Autodesk Inventor part; units mm, degrees
ref_plane "YZ Plane" through (0, 0, 0) normal (1, 0, 0) x (0, 1, 0)
ref_plane "XZ Plane" through (0, 0, 0) normal (0, 1, 0) x (-1, 0, 0)
ref_plane "XY Plane" through (0, 0, 0) normal (0, 0, 1) x (1, 0, 0)
sketch "Sketch1" plane through (0, 0, 0) normal (0, 1, 0) x (-1, 0, 0)
  line L0 (35, 25) -> (-35, 25)
  line L1 (-35, 25) -> (-35, -25)
  line L2 (-35, -25) -> (35, -25)
  line L3 (35, -25) -> (35, 25)
  line L4 (35, 25) -> (-35, -25) construction
  line L5 (-35, 25) -> (35, -25) construction
  line L6 (40, -20) -> (35, -20)
  line L7 (35, -20) -> (35, 20)
  line L8 (35, 20) -> (40, 20)
  line L9 (40, 20) -> (40, -20)
  line L10 (40, -20) -> (35, 20) construction
  line L11 (35, -20) -> (40, 20) construction
  line L12 (-35, -20) -> (-40, -20)
  line L13 (-40, -20) -> (-40, 20)
  line L14 (-40, 20) -> (-35, 20)
  line L15 (-35, 20) -> (-35, -20)
  line L16 (-35, -20) -> (-40, 20) construction
  line L17 (-40, -20) -> (-35, 20) construction
  line L18 (35, 0) -> (0, 0)
  line L19 (37.5, 0) -> (40, 0) construction
  line L20 (-37.5, 0) -> (-35, 0) construction
  point P0 (35, -20)
  point P1 (-35, 20)
  point P2 (-35, -20)
  dimension "d0" = 5
  dimension "d1" = 5
  dimension "d2" = 40
  dimension "d3" = 50
  dimension "d4" = 40
  dimension "d5" = 70
extrude "Extrusion1" add sketch "Sketch1" along normal blind 5
properties part number "Moving Carousel Wall"
Read the model definition and answer for the solid it produces. Units are mm, in the model's axes. A direction names the side the tool comes from. Give positions to 0.01 mm unless a question says otherwise; leave off trailing zeros. Order: outer loops, then holes, each group sorted by start corner. A loop starts at its lowest first (then second) coordinate and runs counter-clockwise, first axis right, second up.
(1) Given pin 1 (1.5 mm diameter, centred on y = 3, z = -23.5, fed in from -X); pin 2 (1.5 mm diameter, centred on x = -38, y = 3, fed in from -Z); pin 3 (1.5 mm diameter, centred on y = 2, z = -22, fed in from +X), each flat-ended and moving along its own axis, determine where each tip first touches the part or whether it passes through.
(2) For faces 1 (the flat face through (37, 2, -20)), 2 (the flat face through (-37, 2, 20)), 3 (the flat face through (35, 2, 23)), 4 (the flat face through (-38, 2, -20)), 5 (the flat face through (1, 5, 0)), determine the directions among +Z, -Z, +X, -X, +Y, -Y from which every point of the face is accessible in a straight line to the end or side of a thin tool.
(3) A straight line is drawn through the part: L1, parallel to X at y = 0.5, z = 22. Find the intervals that lie inside material, in ascending order.
(4) Find section A-A (y = 3.8). Give the vertices of the cut face in (x, z).
Result sheet:
1. pin 1: stops at x = -35
1. pin 2: stops at z = -20
1. pin 3: stops at x = 35
2. face 1: -Z, +X, +Y, -Y
2. face 2: +Z, -X, +Y, -Y
2. face 3: +Z, +X, +Y, -Y
2. face 4: -Z, -X, +Y, -Y
2. face 5: +Z, -Z, +X, -X, +Y
3. L1: x = -35 to 35
4. outline: (-40, -20) - (-35, -20) - (-35, -25) - (35, -25) - (35, -20) - (40, -20) - (40, 20) - (35, 20) - (35, 25) - (-35, 25) - (-35, 20) - (-40, 20) - close
